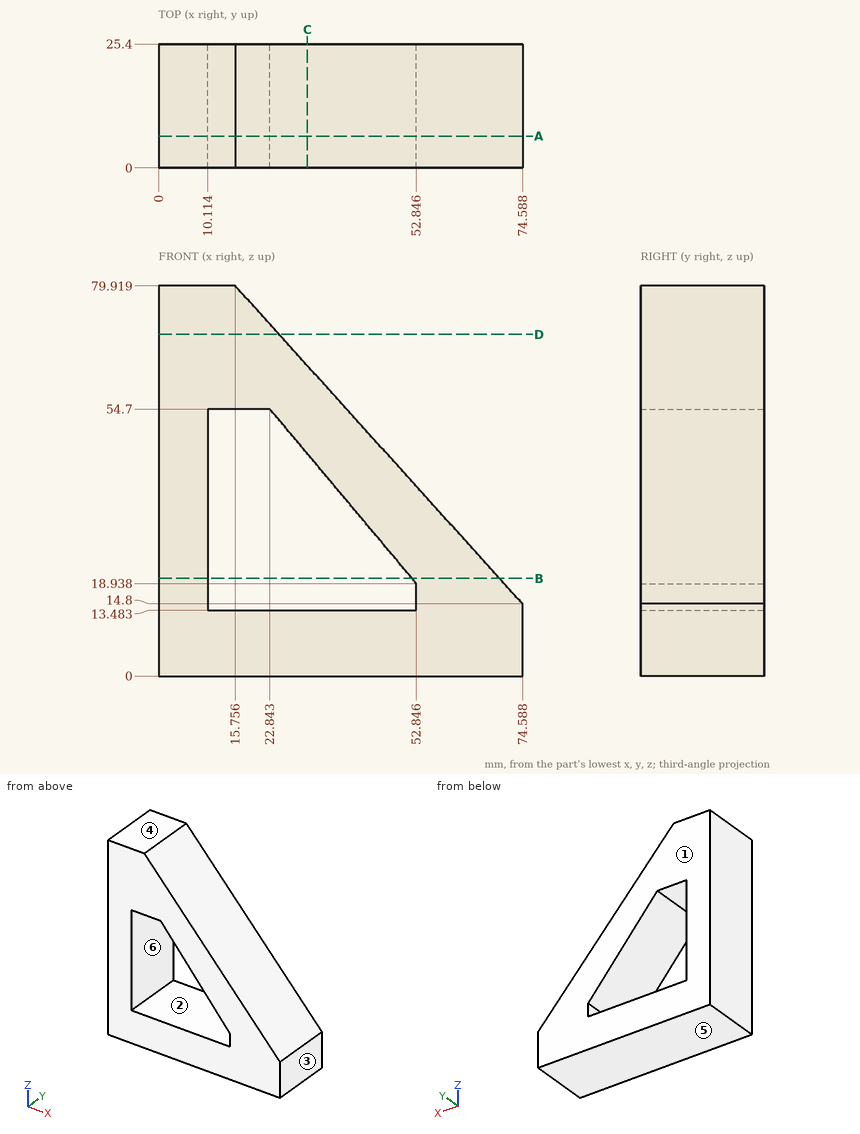
Study the drawing (mm; zero at the part's minimum x, y, z) and answer. A direction names the side the tool comes from. Coordinates: 2 decimals unless noted, no trailing zeros. Order: outer loops, then holes, each group sorted by start corner. A loop starts at its lowest first (then second) coordinate and runs counter-clockwise, first axis right, second up. Notation, with made-up numbers: M 80.25,16 L 126.25,16 A36 cw 126.25,53 Z; hole C 72.25,82 d11. An arc over 180 degrees is marked long. Answer as a JSON object with one key per item and string values. Group by question number.
1. Section D-D on z = 70 is taken. Write down the section's boundary in (x, y).
2. A tool of negligible diameter and unlimited length cuts with its end or side. For the marked faces 1 and 2, from which of +Z, -Z, +X, -X, +Y, -Y can it reach the whole face along a straight path? Write none if from no direction.
3. Determine the mould class of the marked faces 3, 4, 5 and 6 for opening direction Z: released by +Z, released by -Z, zero draft, split by the parting line, or undercut.
4. Section B-B on z = 20 is taken. Write down the section's boundary in (x, y) (1 decimal).
5. Straight lines are drawn through the part: line 1 (Z direction, x = 14, y = 3.5); line 2 (Z direction, x = 26, y = 6.75) (1 decimal); line 3 (X direction, y = 23, z = 52) (1 decimal). For each, find the intervals that lie inside material, in ascending order.
6. Section A-A on y = 6.5 is taken. Write down the section's boundary in (x, z), then the cut area to 3 significant figures.
7. Flat-ended cylindrical pins translate along their axes: P1, Ø8, axis at x = 56, y = 18, coming from the +Z side; P2, Ø4, axis at x = 35.5, y = 17.5, coming from the +Z side. Find the tip coordinate at first contact, or state that the pin passes through.
8. Section C-C on x = 30.5 is taken. Write down the section's boundary in (y, z).
Values follow:
{
 "1": {"outline": "M 0,0 L 24.72,0 L 24.72,25.4 L 0,25.4 Z"},
 "2": {"face 1": "+Z, -Z, +X, -X, +Y", "face 2": "+Y, -Y"},
 "3": {"face 3": "zero draft", "face 4": "released by +Z", "face 5": "released by -Z", "face 6": "undercut"},
 "4": {"outline": "M 0,0 L 10.1,0 L 10.1,25.4 L 0,25.4 Z; M 52,0 L 69.9,0 L 69.9,25.4 L 52,25.4 Z"},
 "5": {"line 1": "0 to 13.48, 54.7 to 79.92", "line 2": "0 to 13.5, 50.9 to 68.6", "line 3": "0 to 10.1, 25.1 to 41"},
 "6": {"outline": "M 0,0 L 74.59,0 L 74.59,14.8 L 15.76,79.92 L 0,79.92 Z; hole M 10.11,13.48 L 52.85,13.48 L 52.85,18.94 L 22.84,54.7 L 10.11,54.7 Z", "area": "2,820 mm2"},
 "7": {"P1": "z = 39.8", "P2": "z = 60.28"},
 "8": {"outline": "M 0,0 L 25.4,0 L 25.4,13.48 L 0,13.48 Z; M 0,45.57 L 25.4,45.57 L 25.4,63.6 L 0,63.6 Z"}
}
